Read the model definition and answer for the solid it produces. Units are mm, in the model's axes. Give positions to 0.01 mm unless a question says otherwise; leave off trailing zeros. Order: outer loops, then holes, each group sorted by start corner. A loop starts at its lowest first (then second) coordinate and runs counter-clockwise, first axis right, second up. Notation, with made-up numbers: (-27, -33.5) - (25, -33.5) arc R25 ccw to (25, -16.5) - close; hole circle Ø11 at (-36.75, 26.5). An arc over 180 degrees is marked (long way). Return JSON: item names as keys, results as strings.
```python
from build123d import *

# Parameters (mm, degrees)
SKETCH_V_W          = 64.58
SKETCH_V_H          = 10
BOSS_EXTRUDE1_DEPTH = 4.75
SKETCH2_R           = 1.75
CUT_EXTRUDE1_DEPTH  = 34.018276757


with BuildPart() as part:
    # Sketch v → Boss-Extrude1 (new body)
    with BuildSketch(Plane(origin=(0, 0, 0), x_dir=(1, 0, 0), z_dir=(0, 1, 0))):
        Rectangle(SKETCH_V_W, SKETCH_V_H)
    extrude(amount=BOSS_EXTRUDE1_DEPTH)

    # Sketch2 → Cut-Extrude1 (cut, through all)
    with BuildSketch(Plane(origin=(0, 4.75, 0), x_dir=(1, 0, 0), z_dir=(0, 1, 0))):
        with Locations(Location((-27.0395, 0, 0), (0, 0, 270))):
            Circle(SKETCH2_R)
        with Locations(Location((27.0305, 0, 0), (0, 0, 270))):
            Circle(SKETCH2_R)
        with Locations(Location((7.5, 0, 0), (0, 0, 270))):
            Circle(SKETCH2_R)
        with Locations(Location((-7.5, 0, 0), (0, 0, 270))):
            Circle(SKETCH2_R)
    extrude(amount=-CUT_EXTRUDE1_DEPTH, mode=Mode.SUBTRACT)


solid = part.part
```
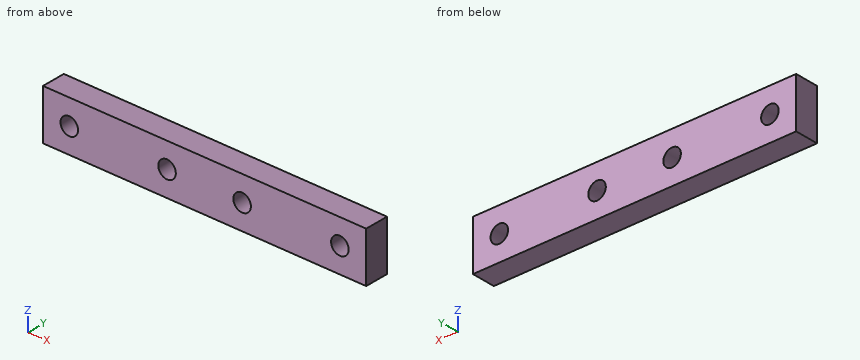
Q1. A cutting plane is placed at A-A (z = 0). Write down the section's boundary in (x, y).
Values:
{"outline": "(-32.29, 0) - (-28.79, 0) - (-28.79, 4.75) - (-32.29, 4.75) - close; (-25.29, 0) - (-9.25, 0) - (-9.25, 4.75) - (-25.29, 4.75) - close; (-5.75, 0) - (5.75, 0) - (5.75, 4.75) - (-5.75, 4.75) - close; (9.25, 0) - (25.28, 0) - (25.28, 4.75) - (9.25, 4.75) - close; (28.78, 0) - (32.29, 0) - (32.29, 4.75) - (28.78, 4.75) - close"}
Q2. A cutting plane is placed at C-C (y = 0.6). Write down the section's boundary in (x, z), and give its area (3 significant figures).
Values:
{"outline": "(-32.29, -5) - (32.29, -5) - (32.29, 5) - (-32.29, 5) - close; hole circle Ø3.5 at (-27.04, 0); hole circle Ø3.5 at (-7.5, 0); hole circle Ø3.5 at (7.5, 0); hole circle Ø3.5 at (27.03, 0)", "area": "607 mm²"}
Q3. Given pin 1 (3 mm diameter, centred on x = 7.5, z = 0, fed in from +Y), flat-ended and moving along its own axis, determine where the tip first touches the part or whether it passes through.
Values:
{"pin 1": "passes through"}
Q4. A cutting plane is placed at B-B (x = 7.5). Write down the section's boundary in (y, z).
Values:
{"outline": "(0, -5) - (4.75, -5) - (4.75, -1.75) - (0, -1.75) - close; (0, 1.75) - (4.75, 1.75) - (4.75, 5) - (0, 5) - close"}
Q5. Consider L1, parallel to X at y = 1.7, z = 0; L2, parallel to X at y = 0.55, z = 0.75; L3, parallel to Z at x = -28, y = 1.35. Determine where each line is inside the solid, lowest interval first.
Values:
{"L1": "x = -32.29 to -28.79, -25.29 to -9.25, -5.75 to 5.75, 9.25 to 25.28, 28.78 to 32.29", "L2": "x = -32.29 to -28.62, -25.46 to -9.08, -5.92 to 5.92, 9.08 to 25.45, 28.61 to 32.29", "L3": "z = -5 to -1.46, 1.46 to 5"}
